The listing builds one solid part. Answer for the finished solid, in the listing's coordinates (mm). A direction names the side the tool comes from. Coordinates: 2 decimals unless noted, no trailing zeros. Loops run counter-clockwise (first coordinate to the right, second up) from the corner with the lowest first, then second, coordinate; pieces in that order, holes last. Notation, with made-up numbers: (73, 41) -> (84, 41) arc R29 ccw to (84, 70) -> close; hole circle Ø11 at (41.25, 75). An arc over 180 degrees is marked (long way). Answer in a Markdown table with one row per item.
Autodesk Inventor part; units mm, degrees
ref_plane "YZ Plane" through (0, 0, 0) normal (1, 0, 0) x (0, 1, 0)
ref_plane "XZ Plane" through (0, 0, 0) normal (0, 1, 0) x (-1, 0, 0)
ref_plane "XY Plane" through (0, 0, 0) normal (0, 0, 1) x (1, 0, 0)
sketch "Sketch1" plane through (0, 0, 0) normal (1, 0, 0) x (0, 1, 0)
  line L0 (0, 0) -> (46, 0)
  line L1 (46, 0) -> (46, -25)
  line L2 (46, -25) -> (0, -25)
  line L3 (0, -25) -> (0, 0)
  dimension "d0" = 46
  dimension "d1" = 25
extrude "Extrusion1" add sketch "Sketch1" along normal blind 138
sketch "Sketch2" plane through (138, 0, 0) normal (1, 0, 0) x (0, 0, -1)
  circle A0 centre (5.5887, 7.0177) radius 3.879
  circle A1 centre (5.5887, 14.0045) radius 2.7237
  point P0 (0, 0)
extrude "Extrusion2" add sketch "Sketch2" along normal blind 10
properties part number "battery1"
Item 1: A cutting plane is placed at A-A, the plane z = -4.5. Determine the outline of the cut face in (x, y).
Findings below:
| item | result |
|---|---|
| outline | (0, 0) -> (138, 0) -> (138, 3.29) -> (148, 3.29) -> (148, 10.74) -> (138, 10.74) -> (138, 11.51) -> (148, 11.51) -> (148, 16.5) -> (138, 16.5) -> (138, 46) -> (0, 46) -> close |
Item 2: Find the intervals of material crossed by probe 1 along X at (y, z) = (32.5, -1.5), in increasing order.
Findings below:
| item | result |
|---|---|
| probe 1 | x = 0 to 138 |
Item 3: Determine the mould class of faces 1 (the face through (142.93, 11.708, -7.053)), 2 (the face through (148, 14, -6)), 3 (the face through (68, 0, -13)) for opening direction Y: +Y half, -Y half, draft (parallel to the pull), parting line (faces both ways), or undercut.
Findings below:
| item | result |
|---|---|
| face 1 | undercut |
| face 2 | draft |
| face 3 | -Y half |
Item 4: A tool of negligible diameter and unlimited length cuts with its end or side. For faces 4 (the face through (68, 23, -25)), 5 (the face through (142.93, 8.503, -9.172)), from which of +Z, -Z, +X, -X, +Y, -Y can it reach the whole face along a straight path? Write none if from no direction.
Findings below:
| item | result |
|---|---|
| face 4 | -Z, +X, -X, +Y, -Y |
| face 5 | +X |
Item 5: A cutting plane is placed at B-B, the plane y = 37. Determine the outline of the cut face in (x, z), plus the area to 3 significant figures.
Findings below:
| item | result |
|---|---|
| outline | (0, -25) -> (138, -25) -> (138, 0) -> (0, 0) -> close |
| area | 3,450 mm2 |
Item 6: A cutting plane is placed at C-C, the plane z = -23.25. Determine the outline of the cut face in (x, y).
Findings below:
| item | result |
|---|---|
| outline | (0, 0) -> (138, 0) -> (138, 46) -> (0, 46) -> close |
